Here's how the part is built. I have some questions about the finished solid (model axes, mm). Face numbers are marked on the shaded views. A direction names the side the tool comes from. Round coordinates to 2 decimals unless told otherwise and drop trailing zeros. Write each loop counter-clockwise with the first axis right and the second up, starting at its lowest first coordinate (ties: lowest second). Pieces come first, ordered by that corner, then holes. Notation, with made-up numbers: (-0.75, 12) -> (12.25, 12) arc R14 cw to (12.25, 25) -> close; hole circle Ø10 at (41.25, 52.5). An arc over 180 degrees is marked (long way). Put each result on its own line as item: value. Start each with the question number.
1. We'd pull the mould along Y, two halves only. Please class the marked faces 6, 7, 8 and 9: +Y half, -Y half, draft (parallel to the pull), parting line (faces both ways), or undercut.
2. Suppose I cut it at A-A (y = 13.5). Please give me the cut outline in (x, z).
3. For pin 1 (5 mm diameter, centred on x = 34, y = 5, fed in from -Z); pin 2 (3 mm diameter, centred on x = 37.5, y = -3, fed in from -Z); pin 3 (1 mm diameter, centred on x = 41, y = 1, fed in from +Z), each with a flat end and sliding along its axis, tell me the tip position at first contact or that it passes through.
4. I need wall thicknesses on probe 1 along X at (y, z) = (0, 13.9); probe 2 along Z at (x, y) = (35.75, 13); probe 3 along Z at (x, y) = (36, -2.5). Which ranges of each line are inside material? Lowest first, please. Write a range as from..to.
5. Suppose I cut it at C-C (z = 6.75). Please give me the cut outline in (x, y).
6. Suppose I cut it at B-B (z = 11). Please give me the cut outline in (x, y).
7. Which directions (+Z, -Z, +X, -X, +Y, -Y) give clear straight access to the entire face, cutting with the end or side of a thin tool? Please do the marked faces 1, 2, 3, 4 and 5.
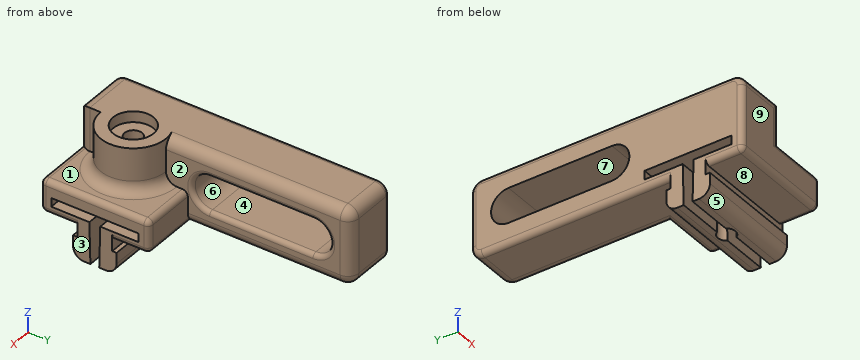
```python
from build123d import *

# Parameters (mm, degrees)
PAD020_DEPTH        = 5
SKETCH037_R         = 3
PAD021_DEPTH        = 4
FILLET013_R         = 1
SKETCH038_W         = 7
SKETCH038_H         = 5
PAD022_DEPTH        = 25
HOLE006_D           = 1.6
HOLE006_CBORE_D     = 3.7
HOLE006_CBORE_DEPTH = 1
POCKET016_DEPTH     = 5.001
POCKET017_DEPTH     = 10.001
FILLET014_R         = 1
FILLET015_R         = 0.5
FILLET017_R         = 0.4
FILLET016_R         = 1


with BuildPart() as part:
    # Sketch035 → Pad020 (new body, symmetric)
    with BuildSketch(Plane.YZ):
        Polygon((-5, 7.5), (-5, 10.5), (5, 10.5), (5, 7.5), (1.6, 7.5), (1.6, 6.5), (2, 6.5), (2, 4.5), (-2, 4.5), (-2, 6.5), (-1.6, 6.5), (-1.6, 7.5), align=None)
    extrude(amount=PAD020_DEPTH, both=True)

    # Sketch037 → Pad021 (join)
    with BuildSketch(Plane(origin=(0, 0, 10.5), x_dir=(0, -1, 0), z_dir=(0, 0, 1))):
        Circle(SKETCH037_R)
    extrude(amount=PAD021_DEPTH)

    # Fillet013
    fillet013_edges = [part.edges().sort_by_distance(p)[0] for p in [
        (0, 3, 10.5),
    ]]
    fillet(fillet013_edges, radius=FILLET013_R)

    # Sketch038 (on DatumPlane) → Pad022 (join)
    with BuildSketch(Plane(origin=(0, -5, 0), x_dir=(0, 0, -1), z_dir=(0, -1, 0))):
        with Locations((-11, -2.5)):
            Rectangle(SKETCH038_W, SKETCH038_H)
    extrude(amount=-PAD022_DEPTH)

    # Hole006 (through all)
    with Locations(Plane(origin=(0, 0, 14.5), x_dir=(0, -1, 0), z_dir=(0, 0, 1))):
        with Locations((0, 0)):
            CounterBoreHole(HOLE006_D / 2, HOLE006_CBORE_D / 2, HOLE006_CBORE_DEPTH)

    # Sketch040 (on DatumPlane) → Pocket016 (cut, through all)
    with BuildSketch(Plane.YZ):
        with BuildLine():
            ThreePointArc((16.5, 9.4), (18.1, 11), (16.5, 12.6))
            Line((7, 12.6), (16.5, 12.6))
            ThreePointArc((7, 12.6), (5.4, 11), (7, 9.4))
            Line((7, 9.4), (16.5, 9.4))
        make_face()
    extrude(amount=-POCKET016_DEPTH, mode=Mode.SUBTRACT)

    # Sketch036 → Pocket017 (cut, through all)
    with BuildSketch(Plane.YZ.offset(5)):
        Polygon((0.5, 8.3), (0.4, 4.3), (-0.4, 4.3), (-0.5, 8.3), (-4, 8.3), (-4, 9.1), (4, 9.1), (4, 8.3), align=None)
    extrude(amount=-POCKET017_DEPTH, mode=Mode.SUBTRACT)

    # Fillet014
    fillet014_edges = [part.edges().sort_by_distance(p)[0] for p in [
        (-2.5, -5, 14.5),
        (0, -5, 12.5),
        (0, 11.5, 14.5),
        (-2.5, 20, 14.5),
        (0, 20, 11),
        (-2.5, 20, 7.5),
        (0, 12.5, 7.5),
    ]]
    fillet(fillet014_edges, radius=FILLET014_R)

    # Fillet015
    fillet015_edges = [part.edges().sort_by_distance(p)[0] for p in [
        (-5, -3.3, 7.5),
        (-5, -5, 10.5),
        (-5, 10.3, 7.5),
        (-5, 7.5, 14.5),
        (-5, -4.707107, 14.207107),
        (-5, 19.707107, 7.792893),
        (-5, 20, 11),
        (-5, 19.707107, 14.207107),
        (5, -3.3, 7.5),
        (5, -5, 9),
        (5, 0, 10.5),
        (5, 5, 9),
        (5, 3.3, 7.5),
        (2.5, 5, 7.5),
        (-0.5, 5, 7.5),
        (2.5, -5, 10.5),
        (-0.5, -5, 10.5),
        (0, -5, 7.5),
        (2.5, 5, 10.5),
    ]]
    fillet(fillet015_edges, radius=FILLET015_R)

    # Fillet017
    fillet017_edges = [part.edges().sort_by_distance(p)[0] for p in [
        (0, 11.75, 12.6),
        (0, 5.4, 11),
        (0, 11.75, 9.4),
        (0, 18.1, 11),
    ]]
    fillet(fillet017_edges, radius=FILLET017_R)

    # Fillet016
    fillet016_edges = [part.edges().sort_by_distance(p)[0] for p in [
        (0, 2, 4.5),
        (0, -2, 4.5),
    ]]
    fillet(fillet016_edges, radius=FILLET016_R)


with BuildPart() as part_1:
    # Body005 placement: moved
    add(part.part.moved(Location((37.45, 0, 0))))


solid = part_1.part
```
Verdict:
1. face 6: undercut
1. face 7: undercut
1. face 8: draft
1. face 9: -Y half
2. outline: (32.45, 8) arc R0.5 ccw to (32.95, 7.5) -> (36.45, 7.5) arc R1 ccw to (37.45, 8.5) -> (37.45, 9) arc R0.4 ccw to (37.05, 9.4) -> (32.45, 9.4) -> close; (32.45, 12.6) -> (37.05, 12.6) arc R0.4 ccw to (37.45, 13) -> (37.45, 13.5) arc R1 ccw to (36.45, 14.5) -> (32.95, 14.5) arc R0.5 ccw to (32.45, 14) -> close
3. pin 1: stops at z = 7.5
3. pin 2: stops at z = 4.63
3. pin 3: stops at z = 10.92
4. probe 1: x = 32.45..35.6, 39.3..40.45
4. probe 2: z = 7.5..9.4, 12.6..14.5
4. probe 3: z = 7.5..8.3, 9.1..14.5
5. outline: (32.45, -1.6) -> (42.45, -1.6) -> (42.45, -0.46) -> (38.1, -0.46) arc R0.8 cw to (36.8, -0.46) -> (32.45, -0.46) -> close; (32.45, 0.46) -> (36.8, 0.46) arc R0.8 cw to (38.1, 0.46) -> (42.45, 0.46) -> (42.45, 1.6) -> (32.45, 1.6) -> close
6. outline: (32.45, -4.5) arc R0.5 ccw to (32.95, -5) -> (36.45, -5) arc R1 ccw to (37.45, -4) -> (37.45, -3.13) arc R3.13 ccw to (37.45, 3.13) -> (37.45, 5) arc R0.4 ccw to (37.05, 5.4) -> (32.45, 5.4) -> close; (32.45, 18.1) -> (37.05, 18.1) arc R0.4 ccw to (37.45, 18.5) -> (37.45, 19) arc R1 ccw to (36.45, 20) -> (32.95, 20) arc R0.5 ccw to (32.45, 19.5) -> close; hole circle Ø1.6 at (37.45, 0)
7. face 1: +Z, +X
7. face 2: +Z, +X, +Y
7. face 3: +Z, -Z, +X, +Y, -Y
7. face 4: +X, -X
7. face 5: -Z, +X, -X, -Y
